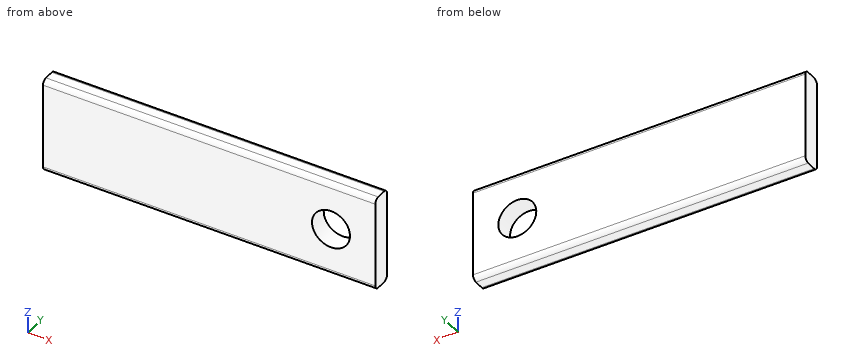
from build123d import *

# Parameters (mm, degrees)
SKETCH_1_W          = 52.5
SKETCH_1_H          = 15
EXTRUDE_1_DEPTH     = 1.5
FILLET_1_R          = 0.75
SKETCH_2_R          = 3
CUT_EXTRUDE_1_DEPTH = 3


with BuildPart() as part:
    # ｽｹｯﾁ1 → ﾎﾞｽ - 押し出し1 (new, symmetric)
    with BuildSketch(Plane(origin=(0, 0, 0), x_dir=(1, 0, 0), z_dir=(0, 1, 0))):
        Rectangle(SKETCH_1_W, SKETCH_1_H)
    extrude(amount=EXTRUDE_1_DEPTH, both=True)

    # ﾌｨﾚｯﾄ1
    fillet_1_edges = [part.edges().sort_by_distance(p)[0] for p in [
        (0, 1.5, 7.5),
        (0, -1.5, 7.5),
        (0, -1.5, -7.5),
        (0, 1.5, -7.5),
    ]]
    fillet(fillet_1_edges, radius=FILLET_1_R)

    # ｽｹｯﾁ2 → ｶｯﾄ - 押し出し1 (cut)
    with BuildSketch(Plane(origin=(0, 1.5, 0), x_dir=(1, 0, 0), z_dir=(0, 1, 0))):
        with Locations(Location((19.25, 0, 0), (0, 0, 270))):
            Circle(SKETCH_2_R)
    extrude(amount=-CUT_EXTRUDE_1_DEPTH, mode=Mode.SUBTRACT)


solid = part.part
Model file for the job. Use its own axes, mm. Round coordinates to 2 decimals unless told otherwise and drop trailing zeros. Order: outer loops, then holes, each group sorted by start corner. A loop starts at its lowest first (then second) coordinate and runs counter-clockwise, first axis right, second up.
(1) Band-saw the part on A-A (x = 19.25). List the corners of the cut face in (y, z), then the cut area to 3 significant figures.
(2) Drill centre lines: line 1 (Z direction, x = 19, y = -0.15); line 2 (X direction, y = 0.2, z = 0); line 3 (Z direction, x = 19, y = 1.15). Where is each one in solid material? Low to high.
(3) Band-saw the part on B-B (z = 0). List the corners of the cut face in (x, y), then the cut area to 4 significant figures.
(4) Band-saw the part on C-C (y = -0.2). List the corners of the cut face in (x, z).
Verdict:
1. outline: (-1.5, -6.75) arc R0.75 ccw to (-0.75, -7.5) - (0.75, -7.5) arc R0.75 ccw to (1.5, -6.75) - (1.5, -3) - (-1.5, -3) - close; (-1.5, 3) - (1.5, 3) - (1.5, 6.75) arc R0.75 ccw to (0.75, 7.5) - (-0.75, 7.5) arc R0.75 ccw to (-1.5, 6.75) - close
1. area: 26.5 mm2
2. line 1: z = -7.5 to -2.99, 2.99 to 7.5
2. line 2: x = -26.25 to 16.25, 22.25 to 26.25
2. line 3: z = -7.38 to -2.99, 2.99 to 7.38
3. outline: (-26.25, -1.5) - (16.25, -1.5) - (16.25, 1.5) - (-26.25, 1.5) - close; (22.25, -1.5) - (26.25, -1.5) - (26.25, 1.5) - (22.25, 1.5) - close
3. area: 139.5 mm2
4. outline: (-26.25, -7.5) - (26.25, -7.5) - (26.25, 7.5) - (-26.25, 7.5) - close; hole circle Ø6 at (19.25, 0)
